Geometry check sheet. Reference: the model listing, model coordinates, mm. Coordinates: 2 decimals unless noted, no trailing zeros. Loops run counter-clockwise (first coordinate to the right, second up) from the corner with the lowest first, then second, coordinate; pieces in that order, holes last. Notation, with made-up numbers: M 28,33 L 66,33 A23 ccw 66,42 Z; hole C 20.5,28.25 d7. An arc over 180 degrees is marked long. Use CSV: the item, a comma, the result in double quotes.
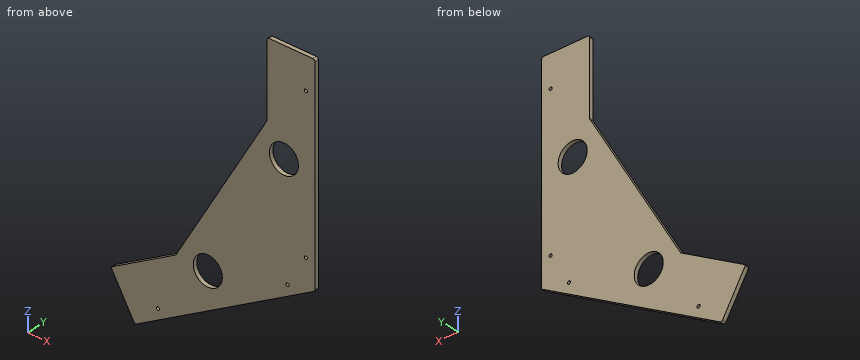
```python
from build123d import *

# Parameters (mm, degrees)
SKETCH1_R           = 23.01875
SKETCH1_R_2         = 2.45745
BOSS_EXTRUDE1_DEPTH = 6.35
FILLET1_R           = 3.175


with BuildPart() as part:
    # Sketch1 → Boss-Extrude1 (new body)
    with BuildSketch(Plane(origin=(0, 0, 0), x_dir=(1, 0, 0), z_dir=(0, 1, 0))):
        Polygon((0, 0), (0, 329.955678842), (-285.75, 494.933518263), (-323.85, 428.942382494), (-220.760110958, 369.423407305), (-76.2, 119.037950379), (-76.2, 0), align=None)
        with Locations((-49.2125, 162.06103122)):
            Circle(SKETCH1_R, mode=Mode.SUBTRACT)
        with Locations((-170.00728, 371.283727469)):
            Circle(SKETCH1_R, mode=Mode.SUBTRACT)
        with Locations((-14.2875, 50.607868786)):
            Circle(SKETCH1_R_2, mode=Mode.SUBTRACT)
        with Locations((-14.2875, 288.082628786)):
            Circle(SKETCH1_R_2, mode=Mode.SUBTRACT)
        with Locations((-43.406875082, 338.518865913)):
            Circle(SKETCH1_R_2, mode=Mode.SUBTRACT)
        with Locations((-249.06605, 457.256245913)):
            Circle(SKETCH1_R_2, mode=Mode.SUBTRACT)
    extrude(amount=BOSS_EXTRUDE1_DEPTH)

    # Fillet1
    fillet1_edges = [part.edges().sort_by_distance(p)[0] for p in [
        (-76.2, 3.175, 0),
        (-76.2, 3.175, -119.037950379),
        (-220.760110958, 3.175, -369.423407305),
        (-323.85, 3.175, -428.942382494),
        (-285.75, 3.175, -494.933518263),
        (0, 3.175, -329.955678842),
        (0, 3.175, 0),
    ]]
    fillet(fillet1_edges, radius=FILLET1_R)


solid = part.part
```
1. Section check B-B, the plane x = -167. Record the cut outline in (y, z).
The answers:
outline,"M 0,-426.37 L 6.35,-426.37 L 6.35,-394.11 L 0,-394.11 Z; M 0,-348.46 L 6.35,-348.46 L 6.35,-276.31 L 0,-276.31 Z"
2. Section check A-A, the plane y = 3.25. Count the separate pieces of the cut face and the enclosed holes in it, plus the area to 3 significant figures.
The answers:
separate pieces,"1"
enclosed holes,"6"
area,"55,600 mm^2"
3. Section check D-D, the plane z = -320.5. Record the cut outline in (x, y), plus the area to 3 significant figures.
The answers:
outline,"M -192.51,0 L 0,0 L 0,6.35 L -192.51,6.35 Z"
area,"1,220 mm^2"
4. Thickness scan on line 1 (Z direction, x = -13, y = 3); line 2 (Z direction, x = -47, y = 5.5); line 3 (X direction, y = 3, z = -33). Record the ranges inside material, lowest first. Write a range as [from, to].
The answers:
line 1,"[-337.46, -290.18], [-285.99, -52.7], [-48.51, 0]"
line 2,"[-357.09, -184.97], [-139.15, 0]"
line 3,"[-76.2, 0]"
5. Gauge pin test, flat ends, axial feed: P1, Ø3, axis at y = 2.5, z = -42.5, coming from the -X side; P2, Ø2, axis at y = 5.5, z = -122.5, coming from the -X side. Record the tip position at first contact, or that the pin passes through.
The answers:
P1,"x = -76.2"
P2,"x = -78.78"
6. Section check C-C, the plane x = -94.5. Record the cut outline in (y, z).
The answers:
outline,"M 0,-384.52 L 6.35,-384.52 L 6.35,-150.73 L 0,-150.73 Z"
